Autodesk Inventor part; units mm, degrees
ref_plane "YZ Plane" through (0, 0, 0) normal (1, 0, 0) x (0, 1, 0)
ref_plane "XZ Plane" through (0, 0, 0) normal (0, 1, 0) x (-1, 0, 0)
ref_plane "XY Plane" through (0, 0, 0) normal (0, 0, 1) x (1, 0, 0)
sketch "Sketch1" plane through (0, 0, 0) normal (0, 0, 1) x (1, 0, 0)
  line L0 (3.175, 0) -> (60.325, 0)
  line L1 (63.5, 3.175) -> (63.5, 22.225)
  line L2 (60.325, 25.4) -> (3.175, 25.4)
  line L3 (0, 22.225) -> (0, 3.175)
  circle A0 centre (6.35, 12.7) radius 2.0701
  line L4 (0, 12.7) -> (63.5, 12.7) construction
  circle A1 centre (31.75, 12.7) radius 2.0701
  circle A2 centre (57.15, 12.7) radius 2.0701
  arc A3 (3.175, 25.4) -> (0, 22.225) centre (3.175, 22.225) ccw
  arc A4 (63.5, 22.225) -> (60.325, 25.4) centre (60.325, 22.225) ccw
  arc A5 (60.325, 0) -> (63.5, 3.175) centre (60.325, 3.175) ccw
  arc A6 (0, 3.175) -> (3.175, 0) centre (3.175, 3.175) ccw
  point P0 (0, 0)
  point P1 (63.5, 25.4)
  point P2 (63.5, 0)
  point P3 (0, 25.4)
  dimension "d0" = 63.5
  dimension "d1" = 25.4
  dimension "d2" = 6.35
  dimension "d3" = 4.1402
  dimension "d6" = 25.4
  dimension "d11" = 3.175
extrude "Extrusion1" add sketch "Sketch1" along normal blind 3.175
properties part number "Spacer 4" material "ABS Plastic"
Input: part model. Units: mm. Frame: model coordinates. Round coordinates to 2 decimals unless told otherwise and drop trailing zeros. Order: outer loops, then holes, each group sorted by start corner. A loop starts at its lowest first (then second) coordinate and runs counter-clockwise, first axis right, second up. Notation, with made-up numbers: (24, -6.75) - (73, -6.75) arc R11 cw to (73, 3.25) - close; hole circle Ø9 at (66, 28.25). An arc over 180 degrees is marked (long way). Use a Markdown table: item, result.
1. Section A-A on z = 1.2. Return the cut outline in (x, y) (3 decimals).
Evaluation:
| item | result |
|---|---|
| outline | (0, 3.175) arc R3.175 ccw to (3.175, 0) - (60.325, 0) arc R3.175 ccw to (63.5, 3.175) - (63.5, 22.225) arc R3.175 ccw to (60.325, 25.4) - (3.175, 25.4) arc R3.175 ccw to (0, 22.225) - close; hole circle Ø4.14 at (6.35, 12.7); hole circle Ø4.14 at (31.75, 12.7); hole circle Ø4.14 at (57.15, 12.7) |
2. Section B-B on x = 6.35. Return the cut outline in (y, z) (3 decimals).
Evaluation:
| item | result |
|---|---|
| outline | (0, 0) - (10.63, 0) - (10.63, 3.175) - (0, 3.175) - close; (14.77, 0) - (25.4, 0) - (25.4, 3.175) - (14.77, 3.175) - close |
3. Material intervals for probe 1 along Y at (x, z) = (57.15, 1.5); probe 2 along X at (y, z) = (11.5, 1.9); probe 3 along Y at (x, z) = (6, 2.95), sorted ascending.
Evaluation:
| item | result |
|---|---|
| probe 1 | 0 to 10.63, 14.77 to 25.4 |
| probe 2 | 0 to 4.66, 8.04 to 30.06, 33.44 to 55.46, 58.84 to 63.5 |
| probe 3 | 0 to 10.66, 14.74 to 25.4 |
4. First-contact query: pin 1 (1.5 mm diameter, centred on y = 12.5, z = 2, fed in from -X). Flat tip, straight axial feed; report the tip coordinate or a pass-through.
Evaluation:
| item | result |
|---|---|
| pin 1 | x = 0 |
5. Mould query, pull axis Y, two halves, no side actions, for faces 1 (the face through (0.91, 24.45, 1.57)), 2 (the face through (29.68, 12.61, 1.57)), 3 (the face through (0.95, 0.91, 1.57)). Classes: +Y half, -Y half, draft (parallel to the pull), parting line (faces both ways), or undercut.
Evaluation:
| item | result |
|---|---|
| face 1 | +Y half |
| face 2 | undercut |
| face 3 | -Y half |
6. Section C-C on y = 12.7. Return the cut outline in (x, z) (3 decimals).
Evaluation:
| item | result |
|---|---|
| outline | (0, 0) - (4.28, 0) - (4.28, 3.175) - (0, 3.175) - close; (8.42, 0) - (29.68, 0) - (29.68, 3.175) - (8.42, 3.175) - close; (33.82, 0) - (55.08, 0) - (55.08, 3.175) - (33.82, 3.175) - close; (59.22, 0) - (63.5, 0) - (63.5, 3.175) - (59.22, 3.175) - close |
